Verification items for the finished model (mm, model axes). Face numbers are marked on the shaded views. A direction names the side the tool comes from. Give positions to 0.01 mm unless a question says otherwise; leave off trailing zeros. Order: outer loops, then holes, each group sorted by start corner. A loop starts at its lowest first (then second) coordinate and runs counter-clockwise, first axis right, second up. Notation, with made-up numbers: (-22, -32.75) -> (-1, -32.75) arc R12 cw to (-1, -14.75) -> close; hole circle Ø9 at (3, 6.5). An arc over 180 degrees is marked (long way). Return JSON: item names as keys, results as strings. Group by question number.
(1) Depth check by flat-ended pin: pin 1 Ø4 at (x, z) = (-50.5, 6) entering from -Y (3 decimals); pin 2 Ø4 at (x, z) = (-12.5, 6.5) entering from -Y; pin 3 Ø3 at (x, z) = (-50.5, 7) entering from +Y (3 decimals). Enter the tip coordinate at first touch or a pass-through.
(2) Cross-section at B-B on x = 1.5. Enter the section's corners in (y, z).
(3) Cross-section at A-A on z = 6.25. Enter the section's corners in (x, y) (3 decimals), then the cut area to 3 significant figures.
(4) Thickness scan on line 1 along X through (y, z) = (4, 11.5); line 2 along X through (y, z) = (0.5, 7.25); line 3 along Y through (x, z) = (-23, 4.5) (3 decimals). Record the ranges inside material, lowest first.
(5) Release check for a two-part mould opening along X. For the marked faces 1, 2 and 3 record: pulls with the +X half, pulls with the -X half, needs draft (parallel to the pull), parting line crosses it, or undercut.
(6) Cross-section at C-C on y = -4.5. Enter the section's corners in (x, z), then the cut area to 3 significant figures.
(7) Tool access check on the marked faces 4, 5, 6, 7 and 8. Record the directions out of +Z, -Z, +X, -X, +Y, -Y that give a thin tool (end or side, any length) a straight path to the whole face; none if there is none.
(8) Cross-section at D-D on x = -25. Enter the section's corners in (y, z) (3 decimals), then the cut area to 3 significant figures.
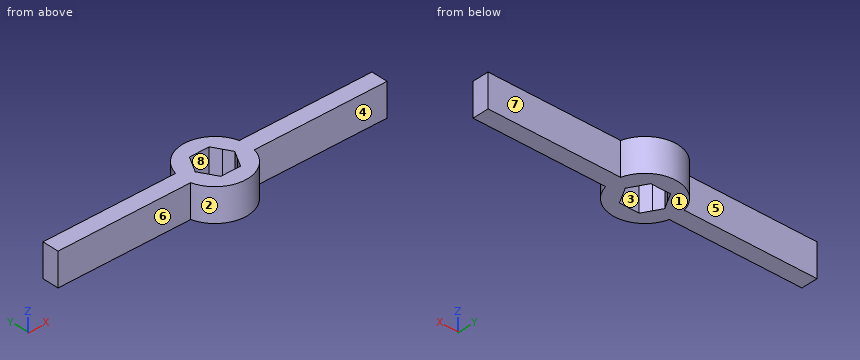
from build123d import *

# Parameters (mm, degrees)
F1_DEPTH = 12.7


with BuildPart() as f1:
    # F0 (on Top) → F1 (new body)
    with BuildSketch(Plane.XY):
        with BuildLine():
            ThreePointArc((-12.296722, -3.175), (-12.7, 0), (-12.296722, 3.175))
            Line((-12.296722, 3.175), (-63.5, 3.175))
            Line((-63.5, 3.175), (-63.5, -3.175))
            Line((-63.5, -3.175), (-12.296722, -3.175))
        make_face()
        with BuildLine():
            Line((-7.625642, 0), (-5.792555, 3.175))
            Line((-5.792555, 3.175), (-12.296722, 3.175))
            ThreePointArc((-12.296722, 3.175), (-12.7, 0), (-12.296722, -3.175))
            Line((-12.296722, -3.175), (-5.792555, -3.175))
            Line((-5.792555, -3.175), (-7.625642, 0))
        make_face()
        with BuildLine():
            Line((-3.812821, 6.604), (3.812821, 6.604))
            Line((3.812821, 6.604), (5.792555, 3.175))
            Line((5.792555, 3.175), (12.296722, 3.175))
            ThreePointArc((12.296722, 3.175), (0, 12.7), (-12.296722, 3.175))
            Line((-12.296722, 3.175), (-5.792555, 3.175))
            Line((-5.792555, 3.175), (-3.812821, 6.604))
        make_face()
        with BuildLine():
            Line((12.296722, 3.175), (5.792555, 3.175))
            Line((5.792555, 3.175), (7.625642, 0))
            Line((7.625642, 0), (5.792555, -3.175))
            Line((5.792555, -3.175), (12.296722, -3.175))
            ThreePointArc((12.296722, -3.175), (12.598777, -1.600255), (12.7, 0))
            ThreePointArc((12.7, 0), (12.598777, 1.600255), (12.296722, 3.175))
        make_face()
        with BuildLine():
            Line((12.296722, -3.175), (5.792555, -3.175))
            Line((5.792555, -3.175), (3.812821, -6.604))
            Line((3.812821, -6.604), (-3.812821, -6.604))
            Line((-3.812821, -6.604), (-5.792555, -3.175))
            Line((-5.792555, -3.175), (-12.296722, -3.175))
            ThreePointArc((-12.296722, -3.175), (0, -12.7), (12.296722, -3.175))
        make_face()
        with BuildLine():
            Line((63.5, 3.175), (12.296722, 3.175))
            ThreePointArc((12.296722, 3.175), (12.598777, 1.600255), (12.7, 0))
            ThreePointArc((12.7, 0), (12.598777, -1.600255), (12.296722, -3.175))
            Line((12.296722, -3.175), (63.5, -3.175))
            Line((63.5, -3.175), (63.5, 3.175))
        make_face()
    extrude(amount=F1_DEPTH)


solid = f1.part
Verdict:
{
 "1": {"pin 1": "y = -3.175", "pin 2": "y = -7.14", "pin 3": "y = 3.175"},
 "2": {"outline": "(-12.61, 0) -> (-6.6, 0) -> (-6.6, 12.7) -> (-12.61, 12.7) -> close; (6.6, 0) -> (12.61, 0) -> (12.61, 12.7) -> (6.6, 12.7) -> close"},
 "3": {"outline": "(-63.5, -3.175) -> (-12.297, -3.175) arc R12.7 ccw to (12.297, -3.175) -> (63.5, -3.175) -> (63.5, 3.175) -> (12.297, 3.175) arc R12.7 ccw to (-12.297, 3.175) -> (-63.5, 3.175) -> close; hole (-7.626, 0) -> (-3.813, -6.604) -> (3.813, -6.604) -> (7.626, 0) -> (3.813, 6.604) -> (-3.813, 6.604) -> close", "area": "1,000 mm²"},
 "4": {"line 1": "-12.05 to -5.32, 5.32 to 12.05", "line 2": "-63.5 to -7.34, 7.34 to 63.5", "line 3": "-3.175 to 3.175"},
 "5": {"face 1": "needs draft", "face 2": "parting line crosses it", "face 3": "undercut"},
 "6": {"outline": "(-11.88, 0) -> (-5.03, 0) -> (-5.03, 12.7) -> (-11.88, 12.7) -> close; (5.03, 0) -> (11.88, 0) -> (11.88, 12.7) -> (5.03, 12.7) -> close", "area": "174 mm²"},
 "7": {"face 4": "+Z, -Z, +X, -Y", "face 5": "+Z, -Z, -X, +Y", "face 6": "+Z, -Z, -X, -Y", "face 7": "+Z, -Z, +X, +Y", "face 8": "+Z, -Z"},
 "8": {"outline": "(-3.175, 0) -> (3.175, 0) -> (3.175, 12.7) -> (-3.175, 12.7) -> close", "area": "80.6 mm²"}
}
